```python
from build123d import *

# Parameters (mm, degrees)
SKETCH1_R           = 3.5
SKETCH1_R_2         = 2
BOSS_EXTRUDE1_DEPTH = 10
FILLET1_R           = 10
SKETCH2_R           = 6.5
CUT_EXTRUDE1_DEPTH  = 5
SKETCH3_R           = 5
CUT_EXTRUDE2_DEPTH  = 4


with BuildPart() as part:
    # Sketch1 → Boss-Extrude1 (new body)
    with BuildSketch(Plane.XY):
        with BuildLine():
            Line((-37.443472345, 17.080292115), (-6.236520765, -7.817020452))
            ThreePointArc((-6.236520765, -7.817020452), (0, -10), (6.236520765, -7.817020452))
            Line((6.236520765, -7.817020452), (37.443472345, 17.080292115))
            ThreePointArc((37.443472345, 17.080292115), (39.84494962, 25.420885127), (32.766081772, 30.443057454))
            Line((32.766081772, 30.443057454), (-32.766081772, 30.443057454))
            ThreePointArc((-32.766081772, 30.443057454), (-39.84494962, 25.420885127), (-37.443472345, 17.080292115))
        make_face()
        Polygon((25.540228058, 20.933819261), (0, 10), (-25.540228058, 20.933819261), align=None, mode=Mode.SUBTRACT)
        Circle(SKETCH1_R, mode=Mode.SUBTRACT)
        with Locations((-32.766081772, 22.943057454)):
            Circle(SKETCH1_R_2, mode=Mode.SUBTRACT)
        with Locations((32.766081772, 22.943057454)):
            Circle(SKETCH1_R_2, mode=Mode.SUBTRACT)
    extrude(amount=BOSS_EXTRUDE1_DEPTH)

    # Fillet1
    fillet1_edges = [part.edges().sort_by_distance(p)[0] for p in [
        (0, 10, 5),
    ]]
    fillet(fillet1_edges, radius=FILLET1_R)

    # Sketch2 → Cut-Extrude1 (cut)
    with BuildSketch(Plane(origin=(0, 0, 0), x_dir=(-1, 0, 0), z_dir=(0, 0, -1))):
        Circle(SKETCH2_R)
    extrude(amount=-CUT_EXTRUDE1_DEPTH, mode=Mode.SUBTRACT)

    # Sketch3 → Cut-Extrude2 (cut)
    with BuildSketch(Plane.XY.offset(10)):
        with Locations((-32.766081772, 22.943057454)):
            Circle(SKETCH3_R)
        with Locations((32.766081772, 22.943057454)):
            Circle(SKETCH3_R)
    extrude(amount=-CUT_EXTRUDE2_DEPTH, mode=Mode.SUBTRACT)


solid = part.part
```
Check sheet for the modelled part. Datum: model origin and axes. Units: mm. A direction names the side the tool comes from. Round coordinates to 2 decimals unless told otherwise and drop trailing zeros. Order: outer loops, then holes, each group sorted by start corner. A loop starts at its lowest first (then second) coordinate and runs counter-clockwise, first axis right, second up. Notation, with made-up numbers: (8.5, -26) -> (53.5, -26) arc R24 cw to (53.5, -10) -> close; hole circle Ø10 at (48.5, 25.5). An arc over 180 degrees is marked (long way). One line per item, written item: value. Start each with the question number.
Q1. Set-up check for faces 1 (the face through (-39.8, 25.54, 4.93)), 2 (the face through (-30.6, 23, 6)), 3 (the face through (-14.587, 16.245, 4.93)): record each of +Z, -Z, +X, -X, +Y, -Y from which the full face is reachable in a straight line by a thin tool's end or side.
Q2. Gauge pin test, flat ends, axial feed: pin 1 Ø5 at (x, y) = (35.5, 25) entering from +Z; pin 2 Ø5 at (y, z) = (6, 1.5) entering from -X; pin 3 Ø6 at (x, y) = (-32.77, 22.94) entering from +Z; pin 4 Ø1 at (y, z) = (-4, 3.5) entering from +X. Record the tip position at first contact, or that the pin passes through.
Q3. Cross-section at B-B (y = 0). Record the boundary of the cut face in (x, z).
Q4. Cross-section at D-D (z = 3.5). Record the boundary of the cut face in (x, y), and give its area (3 significant figures).
Q5. Cross-section at A-A (x = 0). Record the boundary of the cut face in (y, z), and give its area (3 significant figures).
Q6. Cross-section at C-C (x = 9.5). Record the boundary of the cut face in (y, z), and give its area (3 significant figures).
Q7. Thickness scan on line 1 (Y direction, x = 0, z = 6.1); line 2 (Y direction, x = -3, z = 3); line 3 (Z direction, x = 36.5, y = 20). Record the ranges inside material, lowest first.
Completed:
1. face 1: +Z, -Z, -X
1. face 2: +Z
1. face 3: +Z, -Z
2. pin 1: stops at z = 10
2. pin 2: stops at x = -26.69
2. pin 3: stops at z = 6
2. pin 4: stops at x = 11.65
3. outline: (-16.03, 0) -> (-6.5, 0) -> (-6.5, 5) -> (-3.5, 5) -> (-3.5, 10) -> (-16.03, 10) -> close; (3.5, 5) -> (6.5, 5) -> (6.5, 0) -> (16.03, 0) -> (16.03, 10) -> (3.5, 10) -> close
4. outline: (-37.44, 17.08) -> (-6.24, -7.82) arc R10 ccw to (6.24, -7.82) -> (37.44, 17.08) arc R7.5 ccw to (32.77, 30.44) -> (-32.77, 30.44) arc R7.5 ccw to start; hole circle Ø4 at (-32.77, 22.94); hole (-25.54, 20.93) -> (-3.94, 11.68) arc R10 ccw to (3.94, 11.68) -> (25.54, 20.93) -> close; hole circle Ø13 at (0, 0); hole circle Ø4 at (32.77, 22.94)
4. area: 1,710 mm²
5. outline: (-10, 0) -> (-6.5, 0) -> (-6.5, 5) -> (-3.5, 5) -> (-3.5, 10) -> (-10, 10) -> close; (3.5, 5) -> (6.5, 5) -> (6.5, 0) -> (10.88, 0) -> (10.88, 10) -> (3.5, 10) -> close; (20.93, 0) -> (30.44, 0) -> (30.44, 10) -> (20.93, 10) -> close
5. area: 204 mm²
6. outline: (-5.21, 0) -> (14.07, 0) -> (14.07, 10) -> (-5.21, 10) -> close; (20.93, 0) -> (30.44, 0) -> (30.44, 10) -> (20.93, 10) -> close
6. area: 288 mm²
7. line 1: y = -10 to -3.5, 3.5 to 10.88, 20.93 to 30.44
7. line 2: y = -9.54 to -5.77, 5.77 to 11.34, 20.93 to 30.44
7. line 3: z = 0 to 6
